For this review, take the finished solid that the model builds, in its own axes (mm). A direction names the side the tool comes from. Coordinates: 2 decimals unless noted, no trailing zeros. Order: outer loops, then holes, each group sorted by start corner. A loop starts at its lowest first (then second) coordinate and runs counter-clockwise, first axis right, second up. Notation, with made-up numbers: (6.25, 62) -> (25.25, 62) arc R30 ccw to (25.25, 88) -> close; hole circle Ø10 at (5.5, 54). An arc over 180 degrees is marked (long way). Return JSON: item names as keys, results as strings. Group by question number.
Item 1: Take a section at D-D (x = 21). Write out the cut boundary in (y, z), then the cut area to 3 significant figures.
Item 2: Take a section at C-C (y = 7.5). Write out the cut boundary in (x, z).
Item 3: Machinability: for faces 1 (the flat face through (-28, 7, -11)), 2 (the flat face through (28.6, 9.1, -11)), 3 (the flat face through (-12.268, 7, -12)), 4 (the flat face through (-38.5, 7, -13)), which of the approach directions +Z, -Z, +X, -X, +Y, -Y give a long, thin tool a straight path to every point of the face, cutting with its end or side? Answer none if there is none.
Item 4: Take a section at B-B (z = -7). Write out the cut boundary in (x, y), then the cut area to 3 significant figures.
Item 5: Take a section at A-A (x = -30.5). Write out the cut boundary in (y, z), then the cut area to 3 significant figures.
Item 6: For line 1 along X through (y, z) = (9, -10); line 2 along X through (y, z) = (7.5, -13.4); line 3 along Z through (x, y) = (28, 2.5), list the stretches that pass through material, from the lowest coordinate up.
Item 7: Insertion check: pin 1 (1 mm diameter, centred on x = -6, y = 11.5, fed in from +Z); pin 2 (3.5 mm diameter, centred on y = 5, z = -6.5, fed in from -X); pin 3 (7.5 mm diameter, centred on x = -33.5, y = 7, fed in from +Z); pin 4 (4.5 mm diameter, centred on x = -30.5, y = 8, fed in from -Z). Each pin has a flat end and moves straight along its axis. Give the tip position at first contact, or say it passes through.
Item 8: Draft analysis for pull direction Y (two halves, no side actions). For faces 5 (the cylindrical face through (-28.548, 8.434, -13.028)), 6 (the cylindrical face through (32.452, 7.934, -13.028)), 7 (the cylindrical face through (0.407, 7.395, 18.496)), 8 (the flat face through (14, 15, -6)), state which applies: +Y half, -Y half, draft (parallel to the pull), parting line (faces both ways), or undercut.
Autodesk Inventor part; units mm, degrees
ref_plane "YZ Plane" through (0, 0, 0) normal (1, 0, 0) x (0, 1, 0)
ref_plane "XZ Plane" through (0, 0, 0) normal (0, 1, 0) x (-1, 0, 0)
ref_plane "XY Plane" through (0, 0, 0) normal (0, 0, 1) x (1, 0, 0)
sketch "Sketch1" plane through (0, 0, 0) normal (0, 1, 0) x (-1, 0, 0)
  arc A0 (12.2676, -8.6317) -> (-12.2676, -8.6317) centre (0, 0) ccw
  line L0 (-12.2676, -15) -> (-38.5, -15)
  arc A1 (18.5, 0) -> (-18.5, 0) centre (0, 0) ccw
  line L1 (-38.5, -15) -> (-38.5, -11)
  line L2 (-18.5, 0) -> (-18.5, -11)
  line L3 (-38.5, -11) -> (-18.5, -11)
  line L4 (-12.2676, -15) -> (-12.2676, -11)
  line L5 (-12.2676, -11) -> (-12.2676, -8.6317)
  line L6 (38.5, -11) -> (38.5, -15)
  line L7 (38.5, -15) -> (12.2676, -15)
  line L8 (18.5, 0) -> (18.5, -11)
  line L9 (18.5, -11) -> (38.5, -11)
  line L10 (12.2676, -8.6317) -> (12.2676, -15)
  dimension "d0" = 30
  dimension "d1" = 37
  dimension "d2" = 4
  dimension "d3" = 4
  dimension "d4" = 20
  dimension "d5" = 20
extrude "Extrusion1" add sketch "Sketch1" along normal blind 15
hole "Hole1" at (-30.5, 8, -11) direction (0, 0, -1) diameter 4 depth 8 tip angle 118
hole "Hole2" at (30.5, 7.5, -11) direction (0, 0, -1) diameter 4 depth 8 tip angle 118
properties part number "Rohrhalterung"
Findings below:
{
 "1": {"outline": "(0, -15) -> (15, -15) -> (15, -11) -> (0, -11) -> close", "area": "60.0 mm2"},
 "2": {"outline": "(-38.5, -15) -> (-32.44, -15) -> (-32.44, -11) -> (-38.5, -11) -> close; (-28.56, -15) -> (-12.27, -15) -> (-12.27, -8.63) arc R15 cw (long way) to (12.27, -8.63) -> (12.27, -15) -> (28.5, -15) -> (28.5, -11) -> (18.5, -11) -> (18.5, 0) arc R18.5 ccw to (-18.5, 0) -> (-18.5, -11) -> (-28.56, -11) -> close; (32.5, -15) -> (38.5, -15) -> (38.5, -11) -> (32.5, -11) -> close"},
 "3": {"face 1": "+Z, -X, +Y, -Y", "face 2": "+Z, +X, +Y, -Y", "face 3": "-Z, +Y, -Y", "face 4": "+Z, -Z, -X, +Y, -Y"},
 "4": {"outline": "(-18.5, 0) -> (-13.27, 0) -> (-13.27, 15) -> (-18.5, 15) -> close; (13.27, 0) -> (18.5, 0) -> (18.5, 15) -> (13.27, 15) -> close", "area": "157 mm2"},
 "5": {"outline": "(0, -15) -> (6, -15) -> (6, -11) -> (0, -11) -> close; (10, -15) -> (15, -15) -> (15, -11) -> (10, -11) -> close", "area": "44.0 mm2"},
 "6": {"line 1": "x = -18.5 to -12.27, 12.27 to 18.5", "line 2": "x = -38.5 to -32.44, -28.56 to -12.27, 12.27 to 28.5, 32.5 to 38.5", "line 3": "z = -15 to -11"},
 "7": {"pin 1": "stops at z = 17.66", "pin 2": "stops at x = -18.5", "pin 3": "stops at z = -11", "pin 4": "stops at z = -15"},
 "8": {"face 5": "undercut", "face 6": "undercut", "face 7": "draft", "face 8": "+Y half"}
}
